from build123d import *

# Parameters (mm, degrees)
SKETCH1_R           = 5
BOSS_EXTRUDE1_DEPTH = 4


with BuildPart() as part:
    # Sketch1 → Boss-Extrude1 (new body)
    with BuildSketch(Plane.XY):
        Polygon((47, 30), (54.5, 30), (54.5, 25.25), (62.5, 25.25), (62.5, 17.25), (54.5, 17.25), (54.5, 12.5), (47, 12.5), (47, -30), (-81, -30), (-81, 30), align=None)
        with Locations((-36, 0)):
            Circle(SKETCH1_R, mode=Mode.SUBTRACT)
    extrude(amount=BOSS_EXTRUDE1_DEPTH)


solid = part.part
For this review, take the finished solid that the model builds, in its own axes (mm). A direction names the side the tool comes from. Give positions to 0.01 mm unless a question says otherwise; leave off trailing zeros. Loops run counter-clockwise (first coordinate to the right, second up) from the corner with the lowest first, then second, coordinate; pieces in that order, holes last. Notation, with made-up numbers: (34.5, 59.25) - (92.5, 59.25) arc R35 cw to (92.5, 98.25) - close; hole circle Ø2 at (41.25, 23.5). An arc over 180 degrees is marked (long way). Write each question's results on one line, items separated by ' | '.
(1) Take a section at A-A (x = -36). Give the boundary of the cut face in (y, z).
Conclusion:
outline: (-30, 0) - (-5, 0) - (-5, 4) - (-30, 4) - close; (5, 0) - (30, 0) - (30, 4) - (5, 4) - close
(2) For line 1 along Y through (x, z) = (-36, 1.9); line 2 along X through (y, z) = (25.5, 0.85); line 3 along X through (y, z) = (7, 2.15), list the stretches that pass through material, from the lowest coordinate up.
Conclusion:
line 1: -30 to -5, 5 to 30 | line 2: -81 to 54.5 | line 3: -81 to 47
(3) Take a section at D-D (y = -18). Give the boundary of the cut face in (x, z).
Conclusion:
outline: (-81, 0) - (47, 0) - (47, 4) - (-81, 4) - close
(4) For pin 1 Ø5 at (x, y) = (-1, -20) entering from -Z; pin 2 Ø2 at (y, z) = (15.5, 1) entering from +X; pin 3 Ø1.5 at (y, z) = (-23, 1.5) entering from +X; pin 4 Ø2 at (x, z) = (57, 2) entering from +Y, all flat-tipped, find the tip position at first contact; note any pin that passes through.
Conclusion:
pin 1: z = 0 | pin 2: x = 54.5 | pin 3: x = 47 | pin 4: y = 25.25
(5) Take a section at C-C (z = 2.45). Give the boundary of the cut face in (x, y), then the cut area to 3 significant figures.
Conclusion:
outline: (-81, -30) - (47, -30) - (47, 12.5) - (54.5, 12.5) - (54.5, 17.25) - (62.5, 17.25) - (62.5, 25.25) - (54.5, 25.25) - (54.5, 30) - (-81, 30) - close; hole circle Ø10 at (-36, 0) | area: 7,800 mm^2
(6) Draft analysis for pull direction X (two halves, no side actions). For faces 1 (the flat face through (47, -8, 2)), 2 (the flat face through (-81, 0, 2)), 3 (the cylindrical face through (-41, 0, 2)), state which applies: +X half, -X half, draft (parallel to the pull), parting line (faces both ways), or undercut.
Conclusion:
face 1: +X half | face 2: -X half | face 3: undercut
(7) Take a section at B-B (y = 0). Give the boundary of the cut face in (x, z), then the cut area to 3 significant figures.
Conclusion:
outline: (-81, 0) - (-41, 0) - (-41, 4) - (-81, 4) - close; (-31, 0) - (47, 0) - (47, 4) - (-31, 4) - close | area: 472 mm^2
(8) For faces 4 (the flat face through (58, 25.25, 2)), 5 (the flat face through (59, 17.25, 2)), 6 (the flat face through (-8, 0, 0)), list the 3-axis set-ups (+Z, -Z, +X, -X, +Y, -Y) from which the entire face can be reached by the end or side of a thin tool; tool diameter is ignored.
Conclusion:
face 4: +Z, -Z, +X, +Y | face 5: +Z, -Z, +X, -Y | face 6: -Z, +X, -X, +Y, -Y
